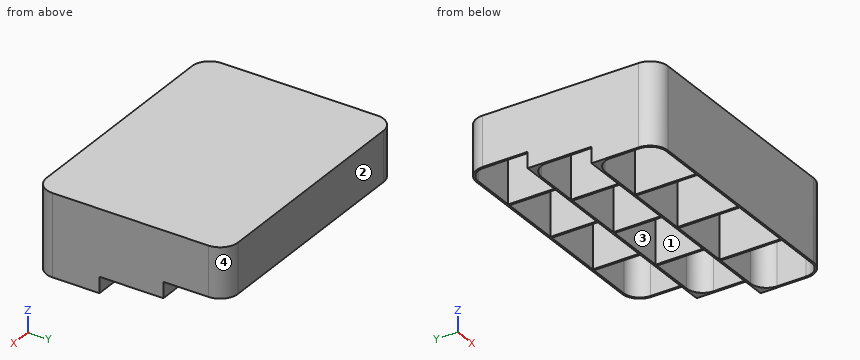
```python
from build123d import *

# Parameters (mm, degrees)
F0_W     = 160
F0_H     = 120
F0_W_2   = 38.2
F0_H_2   = 38.2
F0_W_3   = 38.8
F0_H_3   = 38.8
F1_DEPTH = 50
F2_W     = 160
F2_H     = 120
F3_DEPTH = 1.2
F5_DEPTH = 160.001
F7_DEPTH = 158.8
F8_R     = 10
F9_R     = 11.2
F10_R    = 10


with BuildPart() as f1:
    # F0 (on Top) → F1 (new body)
    with BuildSketch(Plane.XY):
        with Locations((-80, -60)):
            Rectangle(F0_W, F0_H)
        with Locations((-139.7, -99.7)):
            Rectangle(F0_W_2, F0_H_2, mode=Mode.SUBTRACT)
        with Locations((-100, -99.7)):
            Rectangle(F0_W_3, F0_H_2, mode=Mode.SUBTRACT)
        with Locations((-60, -99.7)):
            Rectangle(F0_W_3, F0_H_2, mode=Mode.SUBTRACT)
        with Locations((-20.3, -99.7)):
            Rectangle(F0_W_2, F0_H_2, mode=Mode.SUBTRACT)
        with Locations((-139.7, -60)):
            Rectangle(F0_W_2, F0_H_3, mode=Mode.SUBTRACT)
        with Locations((-100, -60)):
            Rectangle(F0_W_3, F0_H_3, mode=Mode.SUBTRACT)
        with Locations((-139.7, -20.3)):
            Rectangle(F0_W_2, F0_H_2, mode=Mode.SUBTRACT)
        with Locations((-100, -20.3)):
            Rectangle(F0_W_3, F0_H_2, mode=Mode.SUBTRACT)
        with Locations((-60, -60)):
            Rectangle(F0_W_3, F0_H_3, mode=Mode.SUBTRACT)
        with Locations((-20.3, -60)):
            Rectangle(F0_W_2, F0_H_3, mode=Mode.SUBTRACT)
        with Locations((-60, -20.3)):
            Rectangle(F0_W_3, F0_H_2, mode=Mode.SUBTRACT)
        with Locations((-20.3, -20.3)):
            Rectangle(F0_W_2, F0_H_2, mode=Mode.SUBTRACT)
    extrude(amount=F1_DEPTH)

    # F2 (on face) → F3 (join)
    with BuildSketch(Plane.XY.offset(50)):
        with Locations((-80, -60)):
            Rectangle(F2_W, F2_H)
    extrude(amount=F3_DEPTH)

    # F4 (on face) → F5 (cut, through all)
    with BuildSketch(Plane(origin=(-160, 0, 0), x_dir=(0, -1, 0), z_dir=(-1, 0, 0))):
        Polygon((79.4, 0), (79.4, 10), (39.4, 10), (39.4, 20), (0, 20), (0, 0), align=None)
    extrude(amount=-F5_DEPTH, mode=Mode.SUBTRACT)

    # F6 (on face) → F7 (join, through all)
    with BuildSketch(Plane(origin=(-160, 0, 0), x_dir=(0, -1, 0), z_dir=(-1, 0, 0))):
        Polygon((40.6, 50), (40.6, 41.2), (79.4, 41.2), (79.4, 31.2), (118.8, 31.2), (118.8, 50), align=None)
    extrude(amount=-F7_DEPTH)

    # F8
    f8_edges = [f1.edges().sort_by_distance(p)[0] for p in [
        (-1.2, -118.8, 15.6),
        (-1.2, -1.2, 35),
        (-158.8, -118.8, 15.6),
        (-158.8, -1.2, 35),
    ]]
    fillet(f8_edges, radius=F8_R)

    # F9
    f9_edges = [f1.edges().sort_by_distance(p)[0] for p in [
        (-160, 0, 35.6),
        (0, 0, 35.6),
        (0, -120, 25.6),
        (-160, -120, 25.6),
    ]]
    fillet(f9_edges, radius=F9_R)

    # F10
    f10_edges = [f1.edges().sort_by_distance(p)[0] for p in [
        (-158.8, -80.6, 15.6),
        (-158.8, -40.6, 25.6),
        (-1.2, -40.6, 25.6),
        (-1.2, -80.6, 15.6),
    ]]
    fillet(f10_edges, radius=F10_R)


solid = f1.part
```
Read the model definition and answer for the solid it produces. Units are mm, in the model's axes. Face numbers are marked on the shaded views. A direction names the side the tool comes from. Round coordinates to 2 decimals unless told otherwise and drop trailing zeros. Write each loop counter-clockwise with the first axis right and the second up, starting at its lowest first coordinate (ties: lowest second). Pieces come first, ordered by that corner, then holes. Notation, with made-up numbers: (85, 44) - (107, 44) arc R8 cw to (107, 57) - close; hole circle Ø10 at (32, 60). An arc over 180 degrees is marked (long way). Use CSV: the item, a comma, the result in double quotes.
Q1. Find section D-D, the plane y = -28.5. Write down the section's boundary in (x, z), then the cut area to 3 significant figures.
Values:
outline,"(-160, 20) - (-158.8, 20) - (-158.8, 50) - (-120.6, 50) - (-120.6, 20) - (-119.4, 20) - (-119.4, 50) - (-80.6, 50) - (-80.6, 20) - (-79.4, 20) - (-79.4, 50) - (-40.6, 50) - (-40.6, 20) - (-39.4, 20) - (-39.4, 50) - (-1.2, 50) - (-1.2, 20) - (0, 20) - (0, 51.2) - (-160, 51.2) - close"
area,"372 mm²"
Q2. Find section A-A, the plane x = -31. Write down the section's boundary in (y, z).
Values:
outline,"(-120, 0) - (-118.8, 0) - (-118.8, 31.2) - (-80.6, 31.2) - (-80.6, 0) - (-79.4, 0) - (-79.4, 41.2) - (-40.6, 41.2) - (-40.6, 10) - (-39.4, 10) - (-39.4, 50) - (-1.2, 50) - (-1.2, 20) - (0, 20) - (0, 51.2) - (-120, 51.2) - close"
Q3. This flat-tipped pin is pushed along its axis until it touches: pin 1 Ø5 at (x, y) = (-66.5, -101) entering from -Z. Where does it stop, or does it pass through?
Values:
pin 1,"stops at z = 31.2"
Q4. Find section C-C, the plane z = 39. Count the separate pieces of the cut face and the enclosed holes in it, then the cut area to 3 significant figures.
Values:
separate pieces,"1"
enclosed holes,"8"
area,"7,320 mm²"
Q5. Determine the mould class of the marked faces 1 and 2 for opening direction Y: +Y half, -Y half, draft (parallel to the pull), parting line (faces both ways), or undercut.
Values:
face 1,"undercut"
face 2,"+Y half"
Q6. Straight lines are drawn through the part: line 1 along Y through (x, z) = (-18.5, 34); line 2 along X through (y, z) = (-66.5, 30); line 3 along Y through (x, z) = (-47.5, 24). For each, find the intervals that lie inside material, in ascending order.
Values:
line 1,"y = -120 to -79.4, -40.6 to -39.4, -1.2 to 0"
line 2,"x = -160 to -158.8, -120.6 to -119.4, -80.6 to -79.4, -40.6 to -39.4, -1.2 to 0"
line 3,"y = -120 to -118.8, -80.6 to -79.4, -40.6 to -39.4, -1.2 to 0"
Q7. A tool of negligible diameter and unlimited length cuts with its end or side. For the marked faces 3 and 4, from which of +Z, -Z, +X, -X, +Y, -Y can it reach the whole face along a straight path? Write none if from no direction.
Values:
face 3,"-Z"
face 4,"+Z, -Z, +X, +Y"
Q8. Find section B-B, the plane y = -73. Write down the section's boundary in (x, z), then the cut area to 3 significant figures.
Values:
outline,"(-160, 10) - (-158.8, 10) - (-158.8, 41.2) - (-120.6, 41.2) - (-120.6, 10) - (-119.4, 10) - (-119.4, 41.2) - (-80.6, 41.2) - (-80.6, 10) - (-79.4, 10) - (-79.4, 41.2) - (-40.6, 41.2) - (-40.6, 10) - (-39.4, 10) - (-39.4, 41.2) - (-1.2, 41.2) - (-1.2, 10) - (0, 10) - (0, 51.2) - (-160, 51.2) - close"
area,"1,790 mm²"
